The listing builds one solid part. Answer for the finished solid, in the listing's coordinates (mm). Face numbers are marked on the shaded views. A direction names the side the tool comes from. Round coordinates to 2 decimals unless told otherwise and drop trailing zeros. Write each loop counter-clockwise with the first axis right and the second up, starting at its lowest first coordinate (ties: lowest second). Pieces come first, ordered by that corner, then holes.
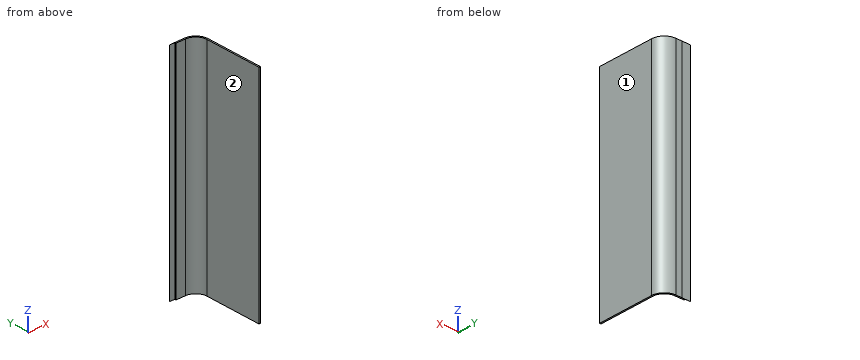
from build123d import *

# Parameters (mm, degrees)
BOSS_EXTRUDE1_DEPTH = 1478.120000035


with BuildPart() as part:
    # Sketch1 → Boss-Extrude1 (new body)
    with BuildSketch(Plane.XY):
        with BuildLine():
            Line((459.721789204, -469.9), (459.721789204, -86.36))
            ThreePointArc((459.721789204, -86.36), (437.403325931, -32.478463274), (383.521789204, -10.16))
            Line((383.521789204, -10.16), (320.021789204, -9.5))
            Line((320.021789204, -9.5), (320.021789204, -0.6))
            Line((320.021789204, -0.6), (284.979491485, -0.6))
            Line((284.979491485, -0.6), (284.979491485, 0))
            Line((284.979491485, 0), (340.976408313, 0))
            Line((340.976408313, 0), (383.5411635, -0.160002177))
            ThreePointArc((383.5411635, -0.160002177), (444.481243206, -25.414245695), (469.721789204, -86.36))
            Line((469.721789204, -86.36), (469.721789204, -469.9))
            Line((469.721789204, -469.9), (459.721789204, -469.9))
        make_face()
    extrude(amount=-BOSS_EXTRUDE1_DEPTH)


solid = part.part
1. Section B-B on x = 301 is taken. Determine the outline of the cut face in (y, z), plus the area to 3 significant figures.
Geometry says:
outline: (-0.6, -1478.12) - (0, -1478.12) - (0, 0) - (-0.6, 0) - close
area: 887 mm2
2. Given pin 1 (1.5 mm diameter, centred on x = 316.5, z = -640.5, fed in from -Y); pin 2 (10 mm diameter, centred on x = 359.5, z = -635, fed in from -Y); pin 3 (2 mm diameter, centred on x = 326.5, z = -818.5, fed in from -Y); pin 4 (4 mm diameter, centred on x = 445, y = -47, fed in from +Z), each flat-ended and moving along its own axis, determine where each tip first touches the part or whether it passes through.
Geometry says:
pin 1: stops at y = -0.6
pin 2: stops at y = -9.96
pin 3: stops at y = -9.58
pin 4: passes through
3. Section C-C on y = -135 is taken. Determine the outline of the cut face in (x, z), plus the area to 3 significant figures.
Geometry says:
outline: (459.72, -1478.12) - (469.72, -1478.12) - (469.72, 0) - (459.72, 0) - close
area: 14,800 mm2
4. Straight lines are drawn through the part: line 1 along X through (y, z) = (-294.5, -158.5); line 2 along Y through (x, z) = (296, -287.5); line 3 along Y through (x, z) = (358.5, -148.5). For each, find the intervals that lie inside material, in ascending order.
Geometry says:
line 1: x = 459.72 to 469.72
line 2: y = -0.6 to 0
line 3: y = -9.9 to -0.07
5. A tool of negligible diameter and unlimited length cuts with its end or side. For the marked faces 1 and 2, from which of +Z, -Z, +X, -X, +Y, -Y can it reach the whole face along a straight path? Write none if from no direction.
Geometry says:
face 1: +Z, -Z, +X, +Y, -Y
face 2: +Z, -Z, -X, -Y
6. Section A-A on z = -876.5 is taken. Determine the outline of the cut face in (x, y), plus the area to 3 significant figures.
Geometry says:
outline: (284.98, -0.6) - (320.02, -0.6) - (320.02, -9.5) - (383.52, -10.16) arc R76.2 cw to (459.72, -86.36) - (459.72, -469.9) - (469.72, -469.9) - (469.72, -86.36) arc R86.2 ccw to (383.54, -0.16) - (340.98, 0) - (284.98, 0) - close
area: 5,750 mm2
